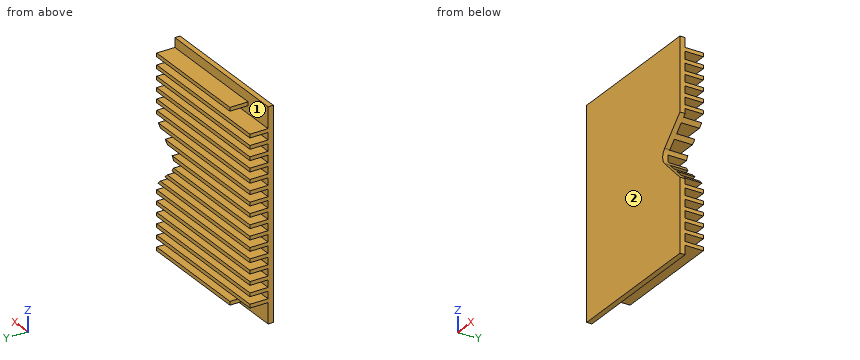
from build123d import *

# Parameters (mm, degrees)
SKETCH_1_W          = 28
SKETCH_1_H          = 40
EXTRUDE_1_DEPTH     = 1
SKETCH_2_W          = 28
SKETCH_2_H          = 0.7
SKETCH_2_W_2        = 22
EXTRUDE_2_DEPTH     = 3.5
CUT_EXTRUDE_1_DEPTH = 25.824383175


with BuildPart() as part:
    # 草图1 → 凸台-拉伸1 (new body)
    with BuildSketch(Plane(origin=(0, 0, 0), x_dir=(1, 0, 0), z_dir=(0, 1, 0))):
        Rectangle(SKETCH_1_W, SKETCH_1_H)
    extrude(amount=EXTRUDE_1_DEPTH)

    # 草图2 → 凸台-拉伸2 (add)
    with BuildSketch(Plane(origin=(0, 1, 0), x_dir=(1, 0, 0), z_dir=(0, 1, 0))):
        with Locations((0, 15.7)):
            Rectangle(SKETCH_2_W, SKETCH_2_H)
        with Locations((0, 13.610934911)):
            Rectangle(SKETCH_2_W, SKETCH_2_H)
        with Locations((0, 11.521869822)):
            Rectangle(SKETCH_2_W, SKETCH_2_H)
        with Locations((0, 9.432804734)):
            Rectangle(SKETCH_2_W, SKETCH_2_H)
        with Locations((0, 7.343739645)):
            Rectangle(SKETCH_2_W, SKETCH_2_H)
        with Locations((0, 5.254674556)):
            Rectangle(SKETCH_2_W, SKETCH_2_H)
        with Locations((0, 3.165609467)):
            Rectangle(SKETCH_2_W, SKETCH_2_H)
        with Locations((0, 1.076544379)):
            Rectangle(SKETCH_2_W, SKETCH_2_H)
        with Locations((0, -1.01252071)):
            Rectangle(SKETCH_2_W, SKETCH_2_H)
        with Locations((0, -3.101585799)):
            Rectangle(SKETCH_2_W, SKETCH_2_H)
        with Locations((0, -5.190650888)):
            Rectangle(SKETCH_2_W, SKETCH_2_H)
        with Locations((0, -7.279715977)):
            Rectangle(SKETCH_2_W, SKETCH_2_H)
        with Locations((0, -9.368781065)):
            Rectangle(SKETCH_2_W, SKETCH_2_H)
        with Locations((0, -11.457846154)):
            Rectangle(SKETCH_2_W, SKETCH_2_H)
        with Locations((0, -13.546911243)):
            Rectangle(SKETCH_2_W, SKETCH_2_H)
        with Locations((0, -15.635976332)):
            Rectangle(SKETCH_2_W, SKETCH_2_H)
        with Locations((3, 17.9)):
            Rectangle(SKETCH_2_W_2, SKETCH_2_H)
        with Locations((3, -17.835976332)):
            Rectangle(SKETCH_2_W_2, SKETCH_2_H)
    extrude(amount=EXTRUDE_2_DEPTH)

    # 草图4 → 切除-拉伸1 (cut, through all)
    with BuildSketch(Plane.XZ):
        with BuildLine():
            Line((9.414213562, -1.414213562), (14, -6))
            Line((14, -6), (14, 6))
            Line((14, 6), (9.414213551, 1.414213551))
            ThreePointArc((9.414213551, 1.414213551), (8.828427125, -8e-09), (9.414213562, -1.414213562))
        make_face()
    extrude(amount=-CUT_EXTRUDE_1_DEPTH, mode=Mode.SUBTRACT)


solid = part.part
Can you work these out from the model? Positions are in its coordinate system, mm. Face numbers are marked on the shaded views. Coordinates: 2 decimals unless noted, no trailing zeros. Write each loop counter-clockwise with the first axis right and the second up, starting at its lowest first coordinate (ties: lowest second). Pieces come first, ordered by that corner, then holes.
Q1. If we mould it in two halves opening along Z, with no side actions, what happens to the marked faces 1 and 2? For each: +Z half, -Z half, draft (parallel to the pull), parting line (faces both ways), or undercut.
Results found:
face 1: undercut
face 2: draft
Q2. Imagine slicing it at A-A, the plane y = 0.5. List the corners of the cut face in (x, z) for me.
Results found:
outline: (-14, -20) - (14, -20) - (14, -6) - (9.41, -1.41) arc R2 cw to (9.41, 1.41) - (14, 6) - (14, 20) - (-14, 20) - close
Q3. Imagine slicing it at C-C, the plane z = 16.5. List the corners of the cut face in (x, y) for me.
Results found:
outline: (-14, 0) - (14, 0) - (14, 1) - (-14, 1) - close
Q4. Imagine slicing it at B-B, the plane y = 3.75. Count the separate pieces of the cut face and the enclosed holes in it, plus the area to 3 significant figures.
Results found:
separate pieces: 18
enclosed holes: 0
area: 332 mm2
Q5. Please list where these lines run through material, in increasing order: L1, parallel to Y at x = -4.75, z = 12; L2, parallel to X at y = 4.35, z = -3.
Results found:
L1: y = 0 to 1
L2: x = -14 to 11
Q6. For P1, Ø0.7, axis at x = 3, z = 6.5, coming from the +Y side; P2, Ø1, axis at x = 2.5, y = 3.5, coming from the +Z side; P3, Ø1, axis at x = 2.5, y = 3, coming from the -Z side, each with a flat end and sliding along its axis, tell me the tip position at first contact or that it passes through.
Results found:
P1: stops at y = 1
P2: stops at z = 18.19
P3: stops at z = -18.25
